```python
from build123d import *

# Parameters (mm, degrees)
F0_R     = 51.778761
F1_DEPTH = 55.626
F2_W     = 30.403304
F2_H     = 28.259708
F3_DEPTH = 110.998


with BuildPart() as f1:
    # F0 (on Front) → F1 (new body)
    with BuildSketch(Plane.XZ):
        Circle(F0_R)
    extrude(amount=F1_DEPTH)

    # F2 (on face) → F3 (cut)
    with BuildSketch(Plane.XZ.offset(55.626)):
        with Locations((-6.091219, 17.017909)):
            Rectangle(F2_W, F2_H)
    extrude(amount=-F3_DEPTH, mode=Mode.SUBTRACT)


solid = f1.part
```
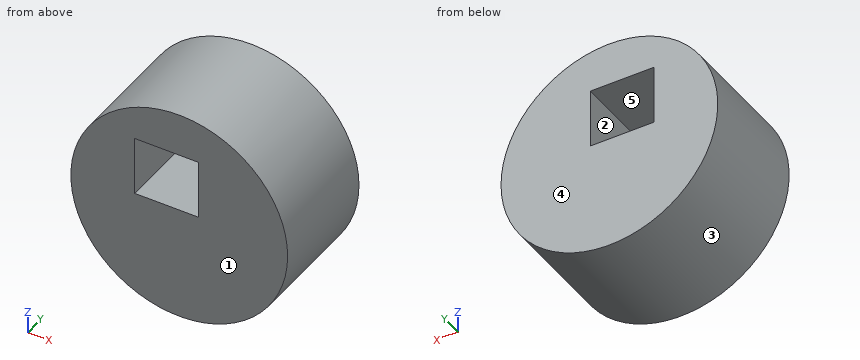
The model under review builds one solid part; all positions refer to its coordinate system, in mm. Face numbers are marked on the shaded views. A direction names the side the tool comes from. Round coordinates to 2 decimals unless told otherwise and drop trailing zeros. Write each loop counter-clockwise with the first axis right and the second up, starting at its lowest first coordinate (ties: lowest second). Pieces come first, ordered by that corner, then holes.
(1) Machinability: for the marked faces 4 and 5, which of the approach directions +Z, -Z, +X, -X, +Y, -Y give a long, thin tool a straight path to every point of the face, cutting with its end or side? Answer none if there is none.
(2) We need section C-C on z = 7. Give the boundary of the cut face in (x, y).
(3) We need section B-B on y = -49. Give the boundary of the cut face in (x, z).
(4) We need section D-D on x = -34.5. Give the boundary of the cut face in (y, z), and give its area (3 significant figures).
(5) Wall thickness on L1, parallel to X at y = -2.5, z = 30.5; L2, parallel to Z at x = 4, y = -48; L3, parallel to X at y = -33, z = 22.5: over which ranges is each line inside the solid? List them lowest first.
(6) We need section A-A on x = 0. Give the boundary of the cut face in (y, z).
(7) Mouldability with a two-part tool opening along Z and no side actions: class the marked faces 1, 2 and 3 as +Z half, -Z half, draft (parallel to the pull), parting line (faces both ways), or undercut.
(8) Insertion check: pin 1 (1 mm diameter, centred on x = 15, y = -11, fed in from +Z); pin 2 (8.5 mm diameter, centred on y = -21, z = 15.5, fed in from -X); pin 3 (4 mm diameter, centred on x = 36.5, y = -27, fed in from +Z). Each pin has a flat end and moves straight along its axis. Give the tip position at first contact, or say it passes through.
Findings below:
1. face 4: +Z, -Z, +X, -X, +Y
1. face 5: +Y, -Y
2. outline: (-51.3, -55.63) - (-21.29, -55.63) - (-21.29, 0) - (-51.3, 0) - close; (9.11, -55.63) - (51.3, -55.63) - (51.3, 0) - (9.11, 0) - close
3. outline: circle Ø103.56 at (0, 0); hole (-21.29, 2.89) - (9.11, 2.89) - (9.11, 31.15) - (-21.29, 31.15) - close
4. outline: (-55.63, -38.61) - (0, -38.61) - (0, 38.61) - (-55.63, 38.61) - close
4. area: 4,300 mm2
5. L1: x = -41.84 to -21.29, 9.11 to 41.84
5. L2: z = -51.62 to 2.89, 31.15 to 51.62
5. L3: x = -46.63 to -21.29, 9.11 to 46.63
6. outline: (-55.63, -51.78) - (0, -51.78) - (0, 2.89) - (-55.63, 2.89) - close; (-55.63, 31.15) - (0, 31.15) - (0, 51.78) - (-55.63, 51.78) - close
7. face 1: draft
7. face 2: undercut
7. face 3: parting line
8. pin 1: stops at z = 49.71
8. pin 2: stops at x = -50.54
8. pin 3: stops at z = 38.61
